from build123d import *
from build123d.topology import SkipClean

# Parameters (mm, degrees)
SKETCH1_R                = 23.241
SKETCH1_R_2              = 9.652
BOSS_EXTRUDE1_DEPTH      = 5.08
BOSS_EXTRUDE2_DEPTH      = 12.7
BOSS_EXTRUDE2_DEPTH_BACK = 17.78
F_1_4_CLEARANCE_HOLE1_D  = 7.14248


with BuildPart() as part:
    # Sketch1 → Boss-Extrude1 (new body)
    with BuildSketch(Plane(origin=(0, 0, 0), x_dir=(1, 0, 0), z_dir=(0, 1, 0))):
        with Locations(Location((0, 0, 0), (0, 0, 270))):
            Circle(SKETCH1_R)
        with Locations(Location((0, 0, 0), (0, 0, 270))):
            Circle(SKETCH1_R_2, mode=Mode.SUBTRACT)
    extrude(amount=BOSS_EXTRUDE1_DEPTH)

    # Sketch2 → Boss-Extrude2 (add, two sides: drawn at the far end of the back side and taken through both)
    with SkipClean():  # the faces are left unmerged after this step: merging them gives an invalid solid
        with BuildSketch(Plane(origin=(0, 5.08, 0), x_dir=(1, 0, 0), z_dir=(0, 1, 0)).offset(-BOSS_EXTRUDE2_DEPTH_BACK)):
            with BuildLine():
                Line((-14.224, 18.379932), (-14.224, 42.291))
                Line((-14.224, 42.291), (-9.652, 42.291))
                Line((-9.652, 42.291), (-9.652, 23.241))
                Line((-9.652, 23.241), (9.652, 23.241))
                Line((9.652, 23.241), (9.652, 42.291))
                Line((9.652, 42.291), (14.224, 42.291))
                Line((14.224, 42.291), (14.224, 18.379932))
                ThreePointArc((14.224, 18.379932), (12.193551, -19.785383), (-22.811972, -4.445))
                Line((-22.811972, -4.445), (-19.567481, -4.445))
                ThreePointArc((-19.567481, -4.445), (20.066, 0), (-19.567481, 4.445))
                Line((-19.567481, 4.445), (-22.811972, 4.445))
                ThreePointArc((-22.811972, 4.445), (-19.785383, 12.193551), (-14.224, 18.379932))
            make_face()
        extrude(amount=BOSS_EXTRUDE2_DEPTH + BOSS_EXTRUDE2_DEPTH_BACK)

    # 1/4 Clearance Hole1 (through all)
    with Locations(Plane(origin=(14.224, 0, 0), x_dir=(0, 0, -1), z_dir=(1, 0, 0))):
        with Locations((32.766, 2.54)):
            Hole(F_1_4_CLEARANCE_HOLE1_D / 2)


solid = part.part
Input: part model. Units: mm. Frame: model coordinates. A direction names the side the tool comes from. Give positions to 0.01 mm unless a question says otherwise; leave off trailing zeros. Order: outer loops, then holes, each group sorted by start corner. A loop starts at its lowest first (then second) coordinate and runs counter-clockwise, first axis right, second up. Notation, with made-up numbers: (57, -22.5) - (104, -22.5) arc R16 ccw to (104, -9.5) - close; hole circle Ø11 at (19, 84.25). An arc over 180 degrees is marked (long way). Answer as a JSON object with one key per item and string values. Group by question number.
Q1. First-contact query: pin 1 Ø1.6 at (x, y) = (-22, -3.5) entering from -Z; pin 2 Ø2.5 at (x, y) = (-21.5, 9) entering from +Z; pin 3 Ø1 at (y, z) = (4, -16.5) entering from -X; pin 4 Ø8 at (x, z) = (-7.5, -23.5) entering from -Y. Flat tips, straight axial feed; report the tip coordinate or a pass-through.
Q2. Mould query, pull axis X, two halves, no side actions, for faces 4 (the face through (-5.87, 2.5, -7.66)), 5 (the face through (9.652, -1, -31)), 6 (the face through (2, 17.78, -22)), 7 (the face through (-14.224, 2, -28)). Classes: pulls with the +X half, pulls with the -X half, needs draft (parallel to the pull), parting line crosses it, or undercut.
Q3. Cut plane C-C, the plane y = 2.54. Output: boundary loops of the cut face in (x, z) (3 decimals).
Q4. Line query: probe 1 along Z at (x, y) = (0, 11); probe 2 along X at (y, z) = (2, 0); probe 3 along X at (y, z) = (-8, 0). Output: solid intervals per line, ascending.
Q5. Cut plane A-A, the plane x = 0. Output: boundary loops of the cut face in (y, z).
Q6. Cut plane D-D, the plane x = -13.5. Output: boundary loops of the cut face in (y, z), then the cut area to 3 significant figures.
Q7. Set-up query: faces 1 (the face through (-21, 11, 4.445)), 2 (the face through (-9.652, -1, -31)), 3 (the face through (4, 0, -9)). Return all of +Z, -Z, +X, -X, +Y, -Y with unobstructed straight access to the full face (end or side cutting, diameter ignored); none if empty.
Q8. Cut plane B-B, the plane z = -26. Output: boundary loops of the cut face in (x, y).
Results:
{
 "1": {"pin 1": "z = -9.52", "pin 2": "z = 11.41", "pin 3": "x = -16.86", "pin 4": "y = -12.7"},
 "2": {"face 4": "undercut", "face 5": "undercut", "face 6": "needs draft", "face 7": "pulls with the -X half"},
 "3": {"outline": "(-22.812, -4.445) arc R23.241 ccw to (-22.243, -6.738) arc R23.241 ccw to (-14.224, -18.38) - (-14.224, -29.195) - (-9.652, -29.195) - (-9.652, -23.241) - (9.652, -23.241) - (9.652, -29.195) - (14.224, -29.195) - (14.224, -18.38) arc R23.241 ccw (long way) to start; (-14.224, -42.291) - (-9.652, -42.291) - (-9.652, -36.337) - (-14.224, -36.337) - close; (9.652, -42.291) - (14.224, -42.291) - (14.224, -36.337) - (9.652, -36.337) - close; hole circle Ø19.304 at (0, 0)"},
 "4": {"probe 1": "-23.24 to -20.07, 20.07 to 23.24", "probe 2": "-23.24 to -9.65, 9.65 to 23.24", "probe 3": "20.07 to 23.24"},
 "5": {"outline": "(-12.7, -23.24) - (17.78, -23.24) - (17.78, -20.07) - (5.08, -20.07) - (5.08, -9.65) - (0, -9.65) - (0, -20.07) - (-12.7, -20.07) - close; (-12.7, 20.07) - (0, 20.07) - (0, 9.65) - (5.08, 9.65) - (5.08, 20.07) - (17.78, 20.07) - (17.78, 23.24) - (-12.7, 23.24) - close"},
 "6": {"outline": "(-12.7, -42.29) - (17.78, -42.29) - (17.78, -14.85) - (5.08, -14.85) - (5.08, 14.85) - (17.78, 14.85) - (17.78, 18.92) - (-12.7, 18.92) - (-12.7, 14.85) - (0, 14.85) - (0, -14.85) - (-12.7, -14.85) - close; hole circle Ø7.14 at (2.54, -32.77)", "area": "1,070 mm^2"},
 "7": {"face 1": "-X, +Y", "face 2": "-Z, +Y, -Y", "face 3": "-Y"},
 "8": {"outline": "(-14.22, -12.7) - (-9.65, -12.7) - (-9.65, 17.78) - (-14.22, 17.78) - close; (9.65, -12.7) - (14.22, -12.7) - (14.22, 17.78) - (9.65, 17.78) - close"}
}
